The model under review builds one solid part; all positions refer to its coordinate system, in mm. Round coordinates to 2 decimals unless told otherwise and drop trailing zeros. Loops run counter-clockwise (first coordinate to the right, second up) from the corner with the lowest first, then second, coordinate; pieces in that order, holes last. Notation, with made-up numbers: M -4.5,60.5 L 23.5,60.5 A11 cw 23.5,79.5 Z; hole C 76.25,59.25 d1. An arc over 180 degrees is marked long. One line per question, with ' | ' between items.
from build123d import *
from build123d.topology import SkipClean

# Parameters (mm, degrees)
SKETCH1_R                = 43.18
SKETCH1_R_2              = 38.1
SKETCH1_R_3              = 36.195
BOSS_EXTRUDE1_DEPTH      = 2.54
BOSS_EXTRUDE2_START      = 4.318
SKETCH2_R                = 43.18
SKETCH2_R_2              = 40.64
BOSS_EXTRUDE2_DEPTH      = 4.318
SKETCH7_W                = 5.08
SKETCH7_H                = 10.16
CUT_EXTRUDE1_DEPTH       = 12.7
SKETCH12_R               = 43.18
SKETCH12_R_2             = 36.195
BOSS_EXTRUDE3_DEPTH      = 12.192
BOSS_EXTRUDE4_REACH      = 99.671
BOSS_EXTRUDE4_END_RADIUS = 43.18
SKETCH13_W               = 43.18
SKETCH13_H               = 24.13
BOSS_EXTRUDE5_DEPTH      = 38.1
SKETCH14_W               = 38.608
SKETCH14_H               = 19.558
CUT_EXTRUDE2_DEPTH       = 35.56
SKETCH17_R               = 3.2385
CUT_EXTRUDE3_DEPTH       = 35.56
CUT_EXTRUDE5_DEPTH       = 88.9
FILLET1_R                = 12.7
SKETCH23_W               = 35.56
SKETCH23_H               = 19.558
CUT_EXTRUDE6_DEPTH       = 50.8


with BuildPart() as part:
    # Sketch1 → Boss-Extrude1 (new body)
    # profile 1 of 2: a face of its own
    with BuildSketch(Plane(origin=(0, 0, 0), x_dir=(1, 0, 0), z_dir=(0, 1, 0))):
        with Locations(Location((0, 0, 0), (0, 0, 270))):
            Circle(SKETCH1_R)
        Circle(SKETCH1_R_2, mode=Mode.SUBTRACT)
    # profile 2 of 2: a face of its own
    with BuildSketch(Plane(origin=(0, 0, 0), x_dir=(1, 0, 0), z_dir=(0, 1, 0))):
        Circle(SKETCH1_R_2)
        with Locations(Location((0, 0, 0), (0, 0, 270))):
            Circle(SKETCH1_R_3, mode=Mode.SUBTRACT)
    extrude(amount=BOSS_EXTRUDE1_DEPTH)

    # Sketch2 → Boss-Extrude2 (add)
    with BuildSketch(Plane.XZ.offset(BOSS_EXTRUDE2_START)):
        with Locations(Location((0, 0, 0), (0, 0, 270))):
            Circle(SKETCH2_R)
        with Locations(Location((0, 0, 0), (0, 0, 270))):
            Circle(SKETCH2_R_2, mode=Mode.SUBTRACT)
    extrude(amount=-BOSS_EXTRUDE2_DEPTH)

    # Sketch3 → Revolve1 (revolve)
    with BuildSketch(Plane.XY, mode=Mode.PRIVATE) as revolve1_sk:
        Polygon((-40.64, -4.318), (-43.18, -4.318), (-43.18, -9.398), (-40.005, -9.398), (-40.005, -6.858), align=None)
    revolve(revolve1_sk.sketch.rotate(Axis((0, 0, 0), (0, 1, 0)), 270), axis=Axis((0, 0, 0), (0, 1, 0)))

    # Sketch7 → Cut-Extrude1 (cut)
    with SkipClean():  # the faces are left unmerged after this step: merging them gives an invalid solid
        with BuildSketch(Plane.XY.offset(43.18)):
            with Locations((-2.54, -5.08)):
                Rectangle(SKETCH7_W, SKETCH7_H)
            with Locations((2.54, -5.08)):
                Rectangle(SKETCH7_W, SKETCH7_H)
        extrude(amount=-CUT_EXTRUDE1_DEPTH, mode=Mode.SUBTRACT)

    # Sketch12 → Boss-Extrude3 (add)
    with SkipClean():  # the faces are left unmerged after this step: merging them gives an invalid solid
        with BuildSketch(Plane(origin=(0, 2.54, 0), x_dir=(1, 0, 0), z_dir=(0, 1, 0))):
            with Locations(Location((0, 0, 0), (0, 0, 263.243672969))):
                Circle(SKETCH12_R)
            with Locations(Location((0, 0, 0), (0, 0, 270))):
                Circle(SKETCH12_R_2, mode=Mode.SUBTRACT)
        extrude(amount=BOSS_EXTRUDE3_DEPTH)

    # Boss-Extrude4: up to this cylinder (the profile starts outside it)
    with SkipClean():  # the faces are left unmerged after this step: merging them gives an invalid solid
        boss_extrude4_end = Plane(origin=(0, 2.667, 0), z_dir=(0, -1, 0)) * Cylinder(BOSS_EXTRUDE4_END_RADIUS, 286.702, mode=Mode.PRIVATE)
        # Sketch8 → Boss-Extrude4 (add, up to the surface)
        with BuildSketch(Plane(origin=(43.18, 0, 0), x_dir=(0, 0, -1), z_dir=(1, 0, 0)), mode=Mode.PRIVATE) as boss_extrude4_sk1:
            Polygon((0.14993237, -9.398), (21.73993237, -9.398), (21.73993237, 14.732), (-21.44006763, 14.732), (-21.44006763, -9.398), align=None)
        boss_extrude4_tool1 = extrude(boss_extrude4_sk1.sketch, amount=-BOSS_EXTRUDE4_REACH, mode=Mode.PRIVATE) - boss_extrude4_end
        add(boss_extrude4_tool1.solids().sort_by_distance((43.18, 2.667, -0.149932))[0])
        add(boss_extrude4_tool1.solids().sort_by_distance((43.18, 2.667, -0.149932))[1])

    # Sketch13 → Boss-Extrude5 (add)
    with SkipClean():  # the faces are left unmerged after this step: merging them gives an invalid solid
        with BuildSketch(Plane(origin=(43.18, 0, 0), x_dir=(0, 0, -1), z_dir=(1, 0, 0))):
            with Locations((0.14993237, 2.667)):
                Rectangle(SKETCH13_W, SKETCH13_H)
        extrude(amount=BOSS_EXTRUDE5_DEPTH)

    # Sketch14 → Cut-Extrude2 (cut)
    with SkipClean():  # the faces are left unmerged after this step: merging them gives an invalid solid
        with BuildSketch(Plane(origin=(81.28, 0, 0), x_dir=(0, 0, -1), z_dir=(1, 0, 0))):
            with Locations((0.14993237, 2.667)):
                Rectangle(SKETCH14_W, SKETCH14_H)
        extrude(amount=-CUT_EXTRUDE2_DEPTH, mode=Mode.SUBTRACT)

    # Sketch17 → Cut-Extrude3 (cut)
    with SkipClean():  # the faces are left unmerged after this step: merging them gives an invalid solid
        with BuildSketch(Plane(origin=(0, 14.732, 0), x_dir=(1, 0, 0), z_dir=(0, 1, 0))):
            with Locations(Location((62.23, 0.14993237, 0), (0, 0, 90))):
                Circle(SKETCH17_R)
        extrude(amount=-CUT_EXTRUDE3_DEPTH, mode=Mode.SUBTRACT)

    # Sketch22 → Cut-Extrude5 (cut)
    with SkipClean():  # the faces are left unmerged after this step: merging them gives an invalid solid
        with BuildSketch(Plane.XY.offset(43.18)):
            Polygon((37.481140591, 14.732), (1.651830342, 3.302), (-49.162594564, 3.302), (-49.162594564, 14.732), align=None)
        extrude(amount=-CUT_EXTRUDE5_DEPTH, mode=Mode.SUBTRACT)

    # Fillet1
    # the kernel refuses this fillet: 12.7 mm, written as the material it adds along each edge
    with BuildSketch(Plane(origin=(1.651830342, 3.302, -31.215644567), x_dir=(0.9526968361956157, 0.30392225700475445, 0), z_dir=(0, 0, -1))) as fillet1_piece_1_section:
        with BuildLine():
            CenterArc((FILLET1_R * 0.155642315474, -FILLET1_R), FILLET1_R, 90, 17.69333606)
            Line((-FILLET1_R * 0.14827994153, -FILLET1_R * 0.0473031638044), (0, 0))
            Line((0, 0), (FILLET1_R * 0.155642315474, 0))
        make_face()
    fillet1_piece_1 = extrude(amount=16.87439239, mode=Mode.PRIVATE)
    fillet1_piece_1 = fillet1_piece_1 & Plane(origin=(0, 3.342340144, 0), x_dir=(-0.11764705883067372, 0, 0.9930554715364556), z_dir=(0, -1, 0)) * Cylinder(43.18, 42, mode=Mode.PRIVATE)
    fillet1_piece_1 = fillet1_piece_1 - Plane(origin=(0, 3.342340144, 0), x_dir=(0, 0, 1), z_dir=(0, -1, 0)) * Cylinder(36.195, 42, mode=Mode.PRIVATE)
    add(fillet1_piece_1)
    with BuildSketch(Plane(origin=(1.651830342, 3.302, 48.090036957), x_dir=(0.9526968361956157, 0.30392225700475445, 0), z_dir=(0, 0, -1))) as fillet1_piece_2_section:
        with BuildLine():
            CenterArc((FILLET1_R * 0.155642315474, -FILLET1_R), FILLET1_R, 90, 17.69333606)
            Line((-FILLET1_R * 0.14827994153, -FILLET1_R * 0.0473031638044), (0, 0))
            Line((0, 0), (FILLET1_R * 0.155642315474, 0))
        make_face()
    fillet1_piece_2 = extrude(amount=16.87439239, mode=Mode.PRIVATE)
    fillet1_piece_2 = fillet1_piece_2 & Plane(origin=(0, 3.342340147, 0), x_dir=(-0.11764705883067372, 0, 0.9930554715364556), z_dir=(0, -1, 0)) * Cylinder(43.18, 42, mode=Mode.PRIVATE)
    fillet1_piece_2 = fillet1_piece_2 - Plane(origin=(0, 3.342340147, 0), x_dir=(0, 0, 1), z_dir=(0, -1, 0)) * Cylinder(36.195, 42, mode=Mode.PRIVATE)
    add(fillet1_piece_2)

    # Sketch23 → Cut-Extrude6 (cut)
    with BuildSketch(Plane.XY.offset(21.44006763)):
        with Locations((63.5, 2.667)):
            Rectangle(SKETCH23_W, SKETCH23_H)
    extrude(amount=-CUT_EXTRUDE6_DEPTH, mode=Mode.SUBTRACT)


solid = part.part
1) Add section A-A on x = 62.23. State the section outline as (y, z) points, then the cut area to 3 significant figures.
Output values:
outline: M -9.4,-21.74 L -7.11,-21.74 L -7.11,-3.39 L -9.4,-3.39 Z; M -9.4,3.09 L -7.11,3.09 L -7.11,21.44 L -9.4,21.44 Z; M 12.45,-21.74 L 14.73,-21.74 L 14.73,-3.39 L 12.45,-3.39 Z; M 12.45,3.09 L 14.73,3.09 L 14.73,21.44 L 12.45,21.44 Z | area: 168 mm²
2) Mouldability with a two-part tool opening along X and no side actions: class faces 1 (the flat face through (5.08, -5, 42)), 2 (the flat face through (-5.08, -5, 42)), 3 (the cylindrical face through (1.66, 3.46, 39.65)), 4 (the flat face through (-38, 3.302, 0)) as +X half, -X half, draft (parallel to the pull), parting line (faces both ways), or undercut.
Output values:
face 1: undercut | face 2: undercut | face 3: -X half | face 4: draft
3) For line 1 (Y direction, x = 49, z = -10.5); line 2 (X direction, y = 0.95, z = 0) (3 decimals); line 3 (Z direction, x = 63.5, y = 13.5), list the stretches that pass through material, from the lowest coordinate up.
Output values:
line 1: y = -9.4 to -7.11, 12.45 to 14.73 | line 2: x = -43.18 to -36.195, 36.195 to 45.72 | line 3: z = -21.74 to -3.13, 2.83 to 21.44
4) Insertion check: P1, Ø3, axis at x = 2.5, z = 41.5, coming from the -Y side; P2, Ø3, axis at x = -12, y = -0.5, coming from the +Z side; P3, Ø5, axis at y = 8.5, z = 23.5, coming from the +X side. Each pin has a flat end and moves straight along its axis. Give the tip position at first contact, or say it passes through.
Output values:
P1: stops at y = 0 | P2: stops at z = 41.88 | P3: stops at x = 45.72
